Design review of the part built by this model. Coordinates are the model's own, in mm. Coordinates: 2 decimals unless noted, no trailing zeros. Loops run counter-clockwise (first coordinate to the right, second up) from the corner with the lowest first, then second, coordinate; pieces in that order, holes last. Notation, with made-up numbers: (66.5, 8.5) -> (113.5, 8.5) arc R9 ccw to (113.5, 23.5) -> close; hole circle Ø8 at (7, 41.5). An arc over 180 degrees is marked (long way). Answer in a Markdown table with one row per item.
```python
from build123d import *

# Parameters (mm, degrees)
SKETCH1_R           = 4.7625
BOSS_EXTRUDE1_DEPTH = 3.175
FILLET1_R           = 25


with BuildPart() as part:
    # Sketch1 → Boss-Extrude1 (new, symmetric)
    # profile 1 of 3: a face of its own
    with BuildSketch(Plane(origin=(0, 0, 0), x_dir=(1, 0, 0), z_dir=(0, 1, 0))):
        with BuildLine():
            Line((-125, -12.5), (-5.17766953, -12.5))
            Line((-5.17766953, -12.5), (-8.838834765, -8.838834765))
            ThreePointArc((-8.838834765, -8.838834765), (-11.548494156, 4.783542905), (0, 12.5))
            Line((0, 12.5), (-125, 12.5))
            ThreePointArc((-125, 12.5), (-137.5, 0), (-125, -12.5))
        make_face()
        with Locations(Location((-125, 0, 0), (0, 0, 270))):
            Circle(SKETCH1_R, mode=Mode.SUBTRACT)
    # profile 2 of 3: a face of its own
    with BuildSketch(Plane(origin=(0, 0, 0), x_dir=(1, 0, 0), z_dir=(0, 1, 0))):
        with BuildLine():
            Line((-5.17766953, -12.5), (0, -12.5))
            ThreePointArc((0, -12.5), (11.548494156, -4.783542905), (8.838834765, 8.838834765))
            ThreePointArc((8.838834765, 8.838834765), (4.783542905, 11.548494156), (0, 12.5))
            ThreePointArc((0, 12.5), (-11.548494156, 4.783542905), (-8.838834765, -8.838834765))
            Line((-8.838834765, -8.838834765), (-5.17766953, -12.5))
        make_face()
        with Locations(Location((0, 0, 0), (0, 0, 270))):
            Circle(SKETCH1_R, mode=Mode.SUBTRACT)
    # profile 3 of 3: a face of its own
    with BuildSketch(Plane(origin=(0, 0, 0), x_dir=(1, 0, 0), z_dir=(0, 1, 0))):
        with BuildLine():
            ThreePointArc((8.838834765, 8.838834765), (11.548494156, -4.783542905), (0, -12.5))
            Line((0, -12.5), (-5.17766953, -12.5))
            Line((-5.17766953, -12.5), (116.161165235, -133.838834765))
            ThreePointArc((116.161165235, -133.838834765), (133.838834765, -133.838834765), (133.838834765, -116.161165235))
            Line((133.838834765, -116.161165235), (8.838834765, 8.838834765))
        make_face()
        with Locations(Location((125, -125, 0), (0, 0, 270))):
            Circle(SKETCH1_R, mode=Mode.SUBTRACT)
        with Locations(Location((79.583029745, -79.583029745, 0), (0, 0, 270))):
            Circle(SKETCH1_R, mode=Mode.SUBTRACT)
    extrude(amount=BOSS_EXTRUDE1_DEPTH, both=True)

    # Fillet1
    fillet1_edges = [part.edges().sort_by_distance(p)[0] for p in [
        (-5.17766953, 0, 12.5),
    ]]
    fillet(fillet1_edges, radius=FILLET1_R)


solid = part.part
```
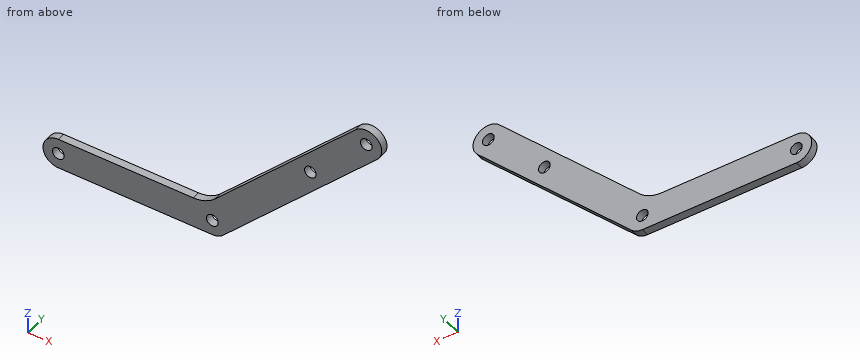
(1) Take a section at A-A on x = 125. Give the boundary of the cut face in (y, z) (1 decimal).
Evaluation:
| item | result |
|---|---|
| outline | (-3.2, 107.3) -> (3.2, 107.3) -> (3.2, 120.2) -> (-3.2, 120.2) -> close; (-3.2, 129.8) -> (3.2, 129.8) -> (3.2, 137.5) -> (-3.2, 137.5) -> close |
(2) Take a section at D-D on y = 0. Give the boundary of the cut face in (x, z) (1 decimal).
Evaluation:
| item | result |
|---|---|
| outline | (-125, -12.5) -> (0, -12.5) arc R12.5 ccw to (8.8, -8.8) -> (133.8, 116.2) arc R12.5 ccw to (116.2, 133.8) -> (2.1, 19.8) arc R25 cw to (-15.5, 12.5) -> (-125, 12.5) arc R12.5 ccw to start; hole circle Ø9.5 at (-125, 0); hole circle Ø9.5 at (0, 0); hole circle Ø9.5 at (79.6, 79.6); hole circle Ø9.5 at (125, 125) |
(3) Take a section at C-C on z = 126.5. Give the boundary of the cut face in (x, y) (3 decimals).
Evaluation:
| item | result |
|---|---|
| outline | (108.822, -3.175) -> (120.48, -3.175) -> (120.48, 3.175) -> (108.822, 3.175) -> close; (129.52, -3.175) -> (137.41, -3.175) -> (137.41, 3.175) -> (129.52, 3.175) -> close |
(4) For pin 1 (3 mm diameter, centred on x = -96, y = 0, fed in from +Z); pin 2 (1.5 mm diameter, centred on y = 2.5, z = 9.5, fed in from -X); pin 3 (1 mm diameter, centred on x = 74, y = 2, fed in from +Z); pin 4 (15 mm diameter, centred on x = 0, z = 0, fed in from -Y) (3 decimals), all flat-tipped, find the tip position at first contact; note any pin that passes through.
Evaluation:
| item | result |
|---|---|
| pin 1 | stops at z = 12.5 |
| pin 2 | stops at x = -133.93 |
| pin 3 | stops at z = 92.18 |
| pin 4 | stops at y = -3.175 |
(5) Take a section at B-B on z = 0. Give the boundary of the cut face in (x, y) (1 decimal).
Evaluation:
| item | result |
|---|---|
| outline | (-137.5, -3.2) -> (-129.8, -3.2) -> (-129.8, 3.2) -> (-137.5, 3.2) -> close; (-120.2, -3.2) -> (-4.8, -3.2) -> (-4.8, 3.2) -> (-120.2, 3.2) -> close; (4.8, -3.2) -> (17.7, -3.2) -> (17.7, 3.2) -> (4.8, 3.2) -> close |
(6) To check wall thickness, follow probe 1 along Z at (x, y) = (-16, -2.5); probe 2 along X at (y, z) = (1.5, -3); probe 3 along X at (y, z) = (2.25, 80). State the ranges of each line that lie inside material, in increasing order.
Evaluation:
| item | result |
|---|---|
| probe 1 | z = -12.5 to 12.5 |
| probe 2 | x = -137.13 to -128.7, -121.3 to -3.7, 3.7 to 14.68 |
| probe 3 | x = 62.32 to 74.84, 84.33 to 97.68 |
